Read the model definition and answer for the solid it produces. Units are mm, in the model's axes. Face numbers are marked on the shaded views. A direction names the side the tool comes from. Coordinates: 2 decimals unless noted, no trailing zeros. Order: outer loops, then holes, each group sorted by start corner. A loop starts at its lowest first (then second) coordinate and runs counter-clockwise, first axis right, second up. Notation, with made-up numbers: (70.5, -6.5) -> (85.5, -6.5) arc R7 cw to (85.5, 5.5) -> close; hole circle Ø6 at (10.25, -3.75). An arc over 180 degrees is marked (long way). Answer as a JSON object with one key per item and string values. Group by question number.
1) A tool of negligible diameter and unlimited length cuts with its end or side. For the marked faces 5, 6, 7, 8 and 9, from which of +Z, -Z, +X, -X, +Y, -Y can it reach the whole face along a straight path? Write none if from no direction.
2) Consider L1, parallel to X at y = 6.5, z = 22; L2, parallel to Z at x = 106, y = 5.25; L3, parallel to X at y = 35.5, z = 15. Determine where each line is inside the solid, lowest interval first.
3) Section D-D on z = 1.5 is taken. Determine the outline of the cut face in (x, y).
4) Section B-B on y = 49.5 is taken. Determine the outline of the cut face in (x, z), and give its area (3 significant figures).
5) Determine the mould class of the marked faces 1, 2, 3 and 4 for opening direction X: released by +X, released by -X, zero draft, split by the parting line, or undercut.
6) Given pin 1 (3.5 mm diameter, centred on x = 36, z = 22, fed in from -Y); pin 2 (19 mm diameter, centred on x = 94.5, z = -16.5, fed in from +Y); pin 3 (4 mm diameter, centred on x = 69.5, z = -20, fed in from -Y); pin 4 (17.5 mm diameter, centred on x = 8.5, z = -0.5, fed in from -Y), each flat-ended and moving along its own axis, determine where each tip first touches the part or whether it passes through.
7) Section C-C on x = 70 is taken. Determine the outline of the cut face in (y, z), and give its area (3 significant figures).
8) Section A-A on x = 19.5 is taken. Determine the outline of the cut face in (y, z), and give its area (3 significant figures).
from build123d import *

# Parameters (mm, degrees)
BOSS_EXTRUDE1_DEPTH  = 32
BOSS_EXTRUDE7_DEPTH  = 22
SKETCH10_R           = 8
CUT_EXTRUDE1_DEPTH   = 22
FILLET1_R            = 3
FILLET2_R            = 3
CUT_EXTRUDE2_DEPTH   = 157.409718368
LPATTERN1_COUNT      = 2
LPATTERN1_PITCH      = 70
LPATTERN1_COUNT_DIR2 = 2
LPATTERN1_PITCH_DIR2 = 44


with BuildPart() as part:
    # Sketch3 → Boss-Extrude1 (new, symmetric)
    with BuildSketch(Plane.XY):
        Polygon((0, 0), (0, 36), (16, 52), (26, 52), (26, 16), (144, 16), (144, 0), align=None)
    extrude(amount=BOSS_EXTRUDE1_DEPTH, both=True)

    # Sketch4 → Boss-Extrude7 (add)
    with BuildSketch(Plane(origin=(144, 0, 0), x_dir=(0, 0, -1), z_dir=(1, 0, 0))):
        with BuildLine():
            Line((-26.927127132, 16), (-14.447851858, 42.761892188))
            ThreePointArc((-14.447851858, 42.761892188), (0.930343347, 51.975931781), (15.207195845, 41.133473752))
            Line((15.207195845, 41.133473752), (26.927127132, 16))
            Line((26.927127132, 16), (-26.927127132, 16))
        make_face()
    extrude(amount=-BOSS_EXTRUDE7_DEPTH)

    # Sketch10 → Cut-Extrude1 (cut)
    with BuildSketch(Plane(origin=(144, 0, 0), x_dir=(0, 0, -1), z_dir=(1, 0, 0))):
        with Locations((0.053072735, 36)):
            Circle(SKETCH10_R)
    extrude(amount=-CUT_EXTRUDE1_DEPTH, mode=Mode.SUBTRACT)

    # Fillet1
    fillet1_edges = [part.edges().sort_by_distance(p)[0] for p in [
        (133, 16, 26.927127132),
    ]]
    fillet(fillet1_edges, radius=FILLET1_R)

    # Fillet2
    fillet2_edges = [part.edges().sort_by_distance(p)[0] for p in [
        (133, 16, -26.927127132),
    ]]
    fillet(fillet2_edges, radius=FILLET2_R)

    # Sketch11 → Cut-Extrude2 (cut, through all)
    with BuildSketch(Plane(origin=(144, 0, 0), x_dir=(0, 0, -1), z_dir=(1, 0, 0))):
        Polygon((-16, -7.593125262), (-16, 7), (-8, 7), (-8, 16), (8, 16), (8, 7), (16, 7), (16, -7.593125262), align=None)
    extrude(amount=-CUT_EXTRUDE2_DEPTH, mode=Mode.SUBTRACT)

    # Sketch13 → Ø1.0mm Dowel Hole1 (revolve, cut)
    with BuildSketch(Plane(origin=(106, 0, 22), x_dir=(0, 0, -1), z_dir=(1, 0, 0))):
        Polygon((0, 0), (0, 11.732050808), (3, 10), (3, 0), align=None)
    f_1_0mm_dowel_hole1 = revolve(axis=Axis((106, -6.35, 22), (0, 1, 0)), mode=Mode.SUBTRACT)

    # LPattern1: 1.0mm Dowel Hole1 2 × 2
    with Locations(*[(-i * LPATTERN1_PITCH, 0, -j * LPATTERN1_PITCH_DIR2) for i in range(LPATTERN1_COUNT) for j in range(LPATTERN1_COUNT_DIR2) if (i, j) != (0, 0)]):
        add(f_1_0mm_dowel_hole1, mode=Mode.SUBTRACT)


solid = part.part
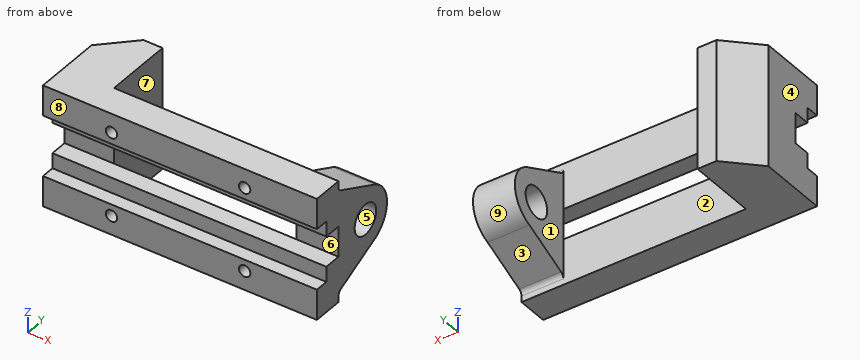
Worked answers:
{
 "1": {"face 5": "+X", "face 6": "+X, -X, -Y", "face 7": "+Z, -Z, +Y", "face 8": "+Z, -Z, +X, -X, -Y", "face 9": "+X, +Y"},
 "2": {"L1": "x = 0 to 33, 39 to 103, 109 to 144", "L2": "z = -32 to -25, -19 to -16, 16 to 19, 25 to 32", "L3": "x = 0 to 26, 122 to 144"},
 "3": {"outline": "(0, 16) -> (26, 16) -> (26, 52) -> (16, 52) -> (0, 36) -> close; (122, 16) -> (144, 16) -> (144, 28.15) -> (122, 28.15) -> close; (122, 43.85) -> (144, 43.85) -> (144, 51.92) -> (122, 51.92) -> close"},
 "4": {"outline": "(13.5, -32) -> (26, -32) -> (26, 32) -> (13.5, 32) -> close; (122, -8.64) -> (144, -8.64) -> (144, 8.53) -> (122, 8.53) -> close", "area": "1,180 mm²"},
 "5": {"face 1": "undercut", "face 2": "undercut", "face 3": "zero draft", "face 4": "released by -X"},
 "6": {"pin 1": "stops at y = 10.72", "pin 2": "stops at y = 16", "pin 3": "stops at y = 0", "pin 4": "stops at y = 7"},
 "7": {"outline": "(0, -32) -> (16, -32) -> (16, -8) -> (7, -8) -> (7, -16) -> (0, -16) -> close; (0, 16) -> (7, 16) -> (7, 8) -> (16, 8) -> (16, 32) -> (0, 32) -> close", "area": "656 mm²"},
 "8": {"outline": "(0, -32) -> (52, -32) -> (52, 32) -> (0, 32) -> (0, 16) -> (7, 16) -> (7, 8) -> (16, 8) -> (16, -8) -> (7, -8) -> (7, -16) -> (0, -16) -> close", "area": "2,960 mm²"}
}
